The model under review builds one solid part; all positions refer to its coordinate system, in mm. A direction names the side the tool comes from. Round coordinates to 2 decimals unless told otherwise and drop trailing zeros. Write each loop counter-clockwise with the first axis right and the second up, starting at its lowest first coordinate (ties: lowest second). Pieces come first, ordered by that corner, then holes.
Item 1: Draft analysis for pull direction X (two halves, no side actions). For faces 3 (the face through (-62.92, -11.89, 0.38)), 4 (the face through (-9, 0, 0)), 5 (the face through (18.444, 12.632, 21.084)), state which applies: +X half, -X half, draft (parallel to the pull), parting line (faces both ways), or undercut.
Item 2: Add section D-D (z = -22). Give the boundary of the cut face in (x, y).
Item 3: To check wall thickness, follow L1, parallel to Z at x = 10, y = 7; L2, parallel to Y at x = -9, z = -19; L3, parallel to X at y = 9.5, z = -9. State the ranges of each line that lie inside material, in increasing order.
Item 4: Add section A-A (x = 26.5). Give the boundary of the cut face in (y, z), plus the area to 3 significant figures.
Item 5: Add section B-B (z = -12.5). Give the boundary of the cut face in (x, y).
Item 6: Clearance check with a flat-ended pin moving along its axis: pin 1 Ø20 at (y, z) = (8.5, -0.5) entering from +X. State where the tip first meets the part, or that it passes through.
Item 7: Add section C-C (y = 12.5). Give the boundary of the cut face in (x, z), plus the area to 3 significant figures.
Item 8: Machinability: for faces 1 (the face through (-18, 11, -27)), 2 (the face through (-0.559, 13, 0)), which of the approach directions +Z, -Z, +X, -X, +Y, -Y give a long, thin tool a straight path to every point of the face, cutting with its end or side? Answer none if there is none.
```python
from build123d import *

# Parameters (mm, degrees)
ESTRUSIONE_ESTRUSIONE1_DEPTH = 27
SMUSSO1_SIZE                 = 10
SMUSSO2_SIZE                 = 5
SCHIZZO2_W                   = 34
SCHIZZO2_H                   = 30
TAGLIO_ESTRUSIONE1_DEPTH     = 86.181546674
SCHIZZO3_R                   = 3
SCHIZZO3_R_2                 = 4
TAGLIO_ESTRUSIONE2_DEPTH     = 94.067963842


with BuildPart() as part:
    # Schizzo1 → Estrusione-Estrusione1 (new, symmetric)
    with BuildSketch(Plane.XY):
        with BuildLine():
            Line((-71.558688457, 25), (33.441311543, 25))
            Line((33.441311543, 25), (33.441311543, 0))
            Line((33.441311543, 0), (-33.441311543, 0))
            ThreePointArc((-33.441311543, 0), (-42.211891736, -2.025659315), (-49.205851182, -7.692307692))
            ThreePointArc((-49.205851182, -7.692307692), (-63.126214368, -11.819696822), (-71.558688457, 0))
            Line((-71.558688457, 0), (-71.558688457, 25))
        make_face()
    extrude(amount=ESTRUSIONE_ESTRUSIONE1_DEPTH, both=True)

    # Smusso1
    smusso1_edges = [part.edges().sort_by_distance(p)[0] for p in [
        (-71.558688457, 25, 0),
    ]]
    chamfer(smusso1_edges, length=SMUSSO1_SIZE)

    # Smusso2
    smusso2_edges = [part.edges().sort_by_distance(p)[0] for p in [
        (33.441311543, 25, 0),
        (33.441311543, 0, 0),
    ]]
    chamfer(smusso2_edges, length=SMUSSO2_SIZE)

    # Schizzo2 → Taglio-Estrusione1 (cut, through all)
    with BuildSketch(Plane(origin=(0, 25, 0), x_dir=(1, 0, 0), z_dir=(0, 1, 0))):
        with Locations((16.441311543, 0)):
            Rectangle(SCHIZZO2_W, SCHIZZO2_H)
    extrude(amount=-TAGLIO_ESTRUSIONE1_DEPTH, mode=Mode.SUBTRACT)

    # Schizzo3 → Taglio-Estrusione2 (cut, through all)
    with BuildSketch(Plane.XY.offset(27)):
        with Locations((21.441311543, 12.5)):
            Circle(SCHIZZO3_R)
        with Locations((-24.558688457, 12.5)):
            Circle(SCHIZZO3_R_2)
    extrude(amount=-TAGLIO_ESTRUSIONE2_DEPTH, mode=Mode.SUBTRACT)


solid = part.part
```
Numbers:
1. face 3: parting line
1. face 4: draft
1. face 5: undercut
2. outline: (-71.56, 0) arc R12.5 ccw to (-49.21, -7.69) arc R20 cw to (-33.44, 0) - (28.44, 0) - (33.44, 5) - (33.44, 20) - (28.44, 25) - (-61.56, 25) - (-71.56, 15) - close; hole circle Ø8 at (-24.56, 12.5); hole circle Ø6 at (21.44, 12.5)
3. L1: z = -27 to -15, 15 to 27
3. L2: y = 0 to 25
3. L3: x = -71.56 to -27.2, -21.91 to -0.56
4. outline: (0, -27) - (25, -27) - (25, -15) - (0, -15) - close; (0, 15) - (25, 15) - (25, 27) - (0, 27) - close
4. area: 600 mm2
5. outline: (-71.56, 0) arc R12.5 ccw to (-49.21, -7.69) arc R20 cw to (-33.44, 0) - (-0.56, 0) - (-0.56, 25) - (-61.56, 25) - (-71.56, 15) - close; hole circle Ø8 at (-24.56, 12.5)
6. pin 1: stops at x = -0.56
7. outline: (-71.56, -27) - (-28.56, -27) - (-28.56, 27) - (-71.56, 27) - close; (-20.56, -27) - (18.44, -27) - (18.44, -15) - (-0.56, -15) - (-0.56, 15) - (18.44, 15) - (18.44, 27) - (-20.56, 27) - close; (24.44, -27) - (33.44, -27) - (33.44, -15) - (24.44, -15) - close; (24.44, 15) - (33.44, 15) - (33.44, 27) - (24.44, 27) - close
7. area: 4,070 mm2
8. face 1: -Z, +X, -X, +Y, -Y
8. face 2: +X, +Y, -Y
